Source: CAD feature listing. Evaluate the final solid. Frame: model axes, mm. Face numbers are marked on the shaded views. A direction names the side the tool comes from. Round coordinates to 2 decimals unless told otherwise and drop trailing zeros. Order: outer loops, then holes, each group sorted by start corner. A loop starts at its lowest first (then second) coordinate and runs counter-clockwise, first axis right, second up. Notation, with made-up numbers: (68.5, -30.5) -> (85.5, -30.5) arc R14 cw to (85.5, -10.5) -> close; hole circle Ø11 at (48.25, 80.25). An arc over 180 degrees is marked (long way). Answer as CSV lines item,"result". Start each with the question number.
(1) Section query C-C (x = 51). Output: boundary loops of the cut face in (y, z).
(2) Line query: line 1 along X through (y, z) = (-9, 4.75); line 2 along Y through (x, z) = (-53, 4); line 3 along Y through (x, z) = (-23.5, 3). Output: solid intervals per line, ascending. Write a range as from..to.
(3) Section query A-A (x = -32). Output: boundary loops of the cut face in (y, z), plus the area to 3 significant figures.
(4) Section query B-B (y = -16.5). Output: boundary loops of the cut face in (x, z), plus the area to 3 significant figures.
(5) Pull-direction query (Y, two-part tool) for the marked faces 1, 2 and 3; classes: +Y half, -Y half, draft (parallel to the pull), parting line (faces both ways), or undercut.
(6) Contact query for flat-ended pins moving along their axis: P1, Ø3, axis at x = 58, z = 9, coming from the -Y side; P2, Ø1.5, axis at x = -30, y = -7.5, coming from the +Z side; P3, Ø0.5, axis at y = 35, z = 6, coming from the +X side. Output: stop coordinate, or through.
(7) Set-up query: the marked faces 4, 5 and 6. Return all of +Z, -Z, +X, -X, +Y, -Y with unobstructed straight access to the full face (end or side cutting, diameter ignored); none if empty.
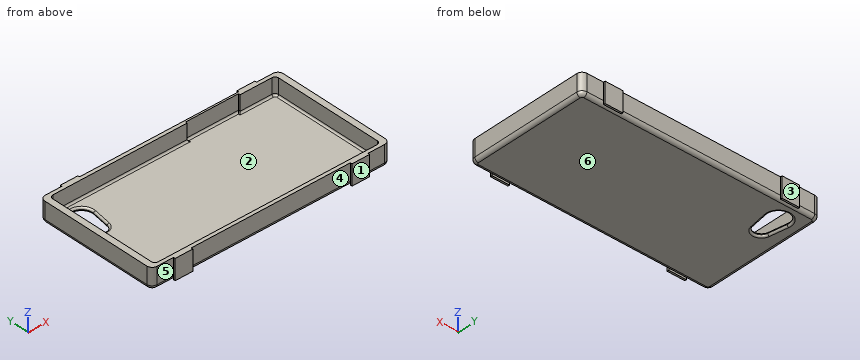
```python
from build123d import *

# Parameters (mm, degrees)
F0_W         = 135
F0_H         = 69
F1_DEPTH     = 11.5
F2_DEPTH     = 2
F3_R         = 2
F4_R         = 2
F5_R         = 1
F6_T1_DEPTH  = 19
F6_T4_ANGLE  = 90
F6_T6_ANGLE  = 90
F6_T8_ANGLE  = 90
F6_T10_ANGLE = 90
F7_W         = 10
F7_H         = 1
F8_DEPTH     = 11.5
F10_DEPTH    = 25
F11_R        = 0.99999


# Not quite as in the source:
# - a fillet or chamfer that OpenCascade refuses, or shapes differently, is made with other operations: its cross-section is extruded or revolved along the edge and cut away or added
# - a fillet or chamfer is up to 0.001 mm smaller than in the source, because OpenCascade refuses the exact size
# - a feature of the source that left no trace in its solid (it failed there, or was rolled back) is left out


with BuildPart() as f1:
    # F0 (on Top) → F1 (new body)
    with BuildSketch(Plane.XY):
        Rectangle(F0_W, F0_H)
        Polygon((-64, -32.5), (-64, 32.5), (14, 32.5), (14, 33.5), (44, 33.5), (44, 32.5), (64, 32.5), (64, -32.5), align=None, mode=Mode.SUBTRACT)
    extrude(amount=F1_DEPTH)

    # F0 (on Top) → F2 (join)
    with BuildSketch(Plane.XY):
        Polygon((14, 32.5), (-64, 32.5), (-64, -32.5), (64, -32.5), (64, 32.5), (44, 32.5), (44, 33.5), (14, 33.5), align=None)
    extrude(amount=F2_DEPTH)

    # F3
    f3_edges = [f1.edges().sort_by_distance(p)[0] for p in [
        (0, 34.5, 0),
        (-67.5, 0, 0),
        (0, -34.5, 0),
        (67.5, 0, 0),
    ]]
    fillet(f3_edges, radius=F3_R)

    # F4
    f4_edges = [f1.edges().sort_by_distance(p)[0] for p in [
        (-64, 32.5, 6.75),
        (64, 32.5, 6.75),
        (64, -32.5, 6.75),
        (-64, -32.5, 6.75),
    ]]
    fillet(f4_edges, radius=F4_R)

    # F5
    f5_edges = [f1.edges().sort_by_distance(p)[0] for p in [
        (-24, 32.5, 2),
        (-63.414214, 31.914214, 2),
        (14, 33, 2),
        (-64, 0, 2),
        (29, 33.5, 2),
        (-63.414214, -31.914214, 2),
        (44, 33, 2),
        (0, -32.5, 2),
        (53, 32.5, 2),
        (63.414214, -31.914214, 2),
        (63.414214, 31.914214, 2),
        (64, 0, 2),
    ]]
    fillet(f5_edges, radius=F5_R)

    # F6: fillet of radius 3 on 4 edges, made by hand

    # F6_s2 → F6_t1 (cut)
    with BuildSketch(Plane.XY):
        with BuildLine():
            ThreePointArc((-64.5, 34.5), (-66.6213203436, 33.6213203436), (-67.5, 31.5))
            Line((-67.5, 31.5), (-67.5, 34.5))
            Line((-67.5, 34.5), (-64.5, 34.5))
        make_face()
        with BuildLine():
            ThreePointArc((-67.5, -31.5), (-66.6213203436, -33.6213203436), (-64.5, -34.5))
            Line((-64.5, -34.5), (-67.5, -34.5))
            Line((-67.5, -34.5), (-67.5, -31.5))
        make_face()
        with BuildLine():
            ThreePointArc((64.5, -34.5), (66.6213203436, -33.6213203436), (67.5, -31.5))
            Line((67.5, -31.5), (67.5, -34.5))
            Line((67.5, -34.5), (64.5, -34.5))
        make_face()
        with BuildLine():
            ThreePointArc((64.5, 34.5), (66.6213203436, 33.6213203436), (67.5, 31.5))
            Line((67.5, 31.5), (67.5, 34.5))
            Line((67.5, 34.5), (64.5, 34.5))
        make_face()
    extrude(amount=F6_T1_DEPTH, mode=Mode.SUBTRACT)

    # F6_s3 → F6_t4 (revolve, cut)
    with BuildSketch(Plane.YZ.offset(64.5)):
        with BuildLine():
            ThreePointArc((32.5, 0), (33.9142135624, 0.5857864376), (34.5, 2))
            Line((34.5, 2), (34.5, 0))
            Line((34.5, 0), (32.5, 0))
        make_face()
    revolve(axis=Axis((64.5, 31.5, 0), (0, 0, -1)), revolution_arc=F6_T4_ANGLE, mode=Mode.SUBTRACT)

    # F6_s5 → F6_t6 (revolve, cut)
    with BuildSketch(Plane.XZ.offset(31.5)):
        with BuildLine():
            ThreePointArc((65.5, 0), (66.9142135624, 0.5857864376), (67.5, 2))
            Line((67.5, 2), (67.5, 0))
            Line((67.5, 0), (65.5, 0))
        make_face()
    revolve(axis=Axis((64.5, -31.5, 0), (0, 0, -1)), revolution_arc=F6_T6_ANGLE, mode=Mode.SUBTRACT)

    # F6_s7 → F6_t8 (revolve, cut)
    with BuildSketch(Plane.YZ.offset(-64.5)):
        with BuildLine():
            ThreePointArc((-32.5, 0), (-33.9142135624, 0.5857864376), (-34.5, 2))
            Line((-34.5, 2), (-34.5, 0))
            Line((-34.5, 0), (-32.5, 0))
        make_face()
    revolve(axis=Axis((-64.5, -31.5, 0), (0, 0, -1)), revolution_arc=F6_T8_ANGLE, mode=Mode.SUBTRACT)

    # F6_s9 → F6_t10 (revolve, cut)
    with BuildSketch(Plane.XZ.offset(-31.5)):
        with BuildLine():
            ThreePointArc((-65.5, 0), (-66.9142135624, 0.5857864376), (-67.5, 2))
            Line((-67.5, 2), (-67.5, 0))
            Line((-67.5, 0), (-65.5, 0))
        make_face()
    revolve(axis=Axis((-64.5, 31.5, 0), (0, 0, -1)), revolution_arc=F6_T10_ANGLE, mode=Mode.SUBTRACT)

    # F7 (on face) → F8 (join, through all)
    with BuildSketch(Plane.XY.offset(11.5)):
        with Locations((-50.1, 35)):
            Rectangle(F7_W, F7_H)
        with Locations((50.1, 35)):
            Rectangle(F7_W, F7_H)
        with Locations((-50.1, -35)):
            Rectangle(F7_W, F7_H)
        with Locations((50.1, -35)):
            Rectangle(F7_W, F7_H)
    extrude(amount=-F8_DEPTH)

    # F9 (on face) → F10 (cut)
    with BuildSketch(Plane.XY.offset(2)):
        with BuildLine():
            Line((-50.2595349939, 11.8031518124), (-48.5794111489, 22.0270520794))
            ThreePointArc((-48.5794111489, 22.0270520794), (-54.5, 29), (-60.4205888511, 22.0270520794))
            Line((-60.4205888511, 22.0270520794), (-58.7404650061, 11.8031518124))
            ThreePointArc((-58.7404650061, 11.8031518124), (-54.5, 8.2026588611), (-50.2595349939, 11.8031518124))
        make_face()
    extrude(amount=-F10_DEPTH, mode=Mode.SUBTRACT)

    # F11 (radius 1 in the source; OpenCascade refuses exactly that, so slightly less here)
    f11_edges = [f1.edges().sort_by_distance(p)[0] for p in [
        (-54.5, 29, 2),
        (-49.419473, 16.915102, 0),
        (-54.5, 8.202659, 2),
        (-49.419473, 16.915102, 2),
        (-59.580527, 16.915102, 2),
        (-54.5, 8.202659, 0),
        (-54.5, 29, 0),
        (-59.580527, 16.915102, 0),
    ]]
    fillet(f11_edges, radius=F11_R)


solid = f1.part
```
Answer block:
1,outline,"(-35.5, 0) -> (-34.5, 0) -> (-34.5, 2) arc R2 ccw to (-32.5, 0) -> (32.5, 0) arc R2 ccw to (34.5, 2) -> (34.5, 0) -> (35.5, 0) -> (35.5, 11.5) -> (32.5, 11.5) -> (32.5, 3) arc R1 cw to (31.5, 2) -> (-31.5, 2) arc R1 cw to (-32.5, 3) -> (-32.5, 11.5) -> (-35.5, 11.5) -> close"
2,line 1,"-67.5..-64, 64..67.5"
2,line 2,"-35.5..-32.5, 32.5..35.5"
2,line 3,"-34.5..-32.5, 32.5..34.5"
3,outline,"(-34.5, 2) arc R2 ccw to (-32.5, 0) -> (32.5, 0) arc R2 ccw to (34.5, 2) -> (34.5, 11.5) -> (32.5, 11.5) -> (32.5, 3) arc R1 cw to (31.5, 2) -> (-31.5, 2) arc R1 cw to (-32.5, 3) -> (-32.5, 11.5) -> (-34.5, 11.5) -> close"
3,area,"175 mm2"
4,outline,"(-67.5, 2) arc R2 ccw to (-65.5, 0) -> (65.5, 0) arc R2 ccw to (67.5, 2) -> (67.5, 11.5) -> (64, 11.5) -> (64, 3) arc R1 cw to (63, 2) -> (-63, 2) arc R1 cw to (-64, 3) -> (-64, 11.5) -> (-67.5, 11.5) -> close"
4,area,"335 mm2"
5,face 1,"-Y half"
5,face 2,"undercut"
5,face 3,"+Y half"
6,P1,"y = -34.5"
6,P2,"z = 2"
6,P3,"x = 55.1"
7,face 4,"+Z, -Z, -Y"
7,face 5,"+Z, -Z, -X, -Y"
7,face 6,"-Z, +X, -X, +Y, -Y"
